Read the model definition and answer for the solid it produces. Units are mm, in the model's axes. A direction names the side the tool comes from. Coordinates: 2 decimals unless noted, no trailing zeros. Loops run counter-clockwise (first coordinate to the right, second up) from the corner with the lowest first, then second, coordinate; pieces in that order, holes last.
Autodesk Inventor part; units mm, degrees
ref_plane "YZ Plane" through (0, 0, 0) normal (1, 0, 0) x (0, 1, 0)
ref_plane "XZ Plane" through (0, 0, 0) normal (0, 1, 0) x (-1, 0, 0)
ref_plane "XY Plane" through (0, 0, 0) normal (0, 0, 1) x (1, 0, 0)
sketch "Sketch1" plane through (0, 0, 0) normal (0, 0, 1) x (1, 0, 0)
  line L0 (0, 0) -> (45.72, 0)
  line L1 (45.72, 0) -> (45.72, 34.29)
  line L2 (0, 0) -> (0, 82.169) construction
  line L3 (45.72, 34.29) -> (0, 82.169)
  line L4 (0, 0) -> (-45.72, 0)
  line L5 (-45.72, 0) -> (-45.72, 34.29)
  line L6 (-45.72, 34.29) -> (0, 82.169)
  dimension "d0" = 82.169
  dimension "d1" = 45.72
  dimension "d2" = 34.29
extrude "Extrusion1" add sketch "Sketch1" against normal blind 3.175
sketch "Sketch2" plane through (0, 0, 0) normal (0, 0, 1) x (1, 0, 0)
  line L0 (-45.72, 0) -> (-45.72, 34.29)
  line L1 (-45.72, 0) -> (45.72, 0)
  line L2 (45.72, 0) -> (45.72, 3.175)
  line L3 (45.72, 3.175) -> (-45.72, 3.175)
  line L4 (-45.72, 3.175) -> (-45.72, 0)
  point P0 (0, 0)
  dimension "d5" = 3.175
extrude "Extrusion2" add sketch "Sketch2" along normal blind 20.32
sketch "Sketch3" plane through (0, 0, 0) normal (0, 0, 1) x (1, 0, 0)
  circle A0 centre (0, 34.925) radius 15.113
  line L0 (-45.72, 0) -> (45.72, 0)
  point P0 (0, 0)
  dimension "d8" = 30.226
  dimension "d9" = 34.925
extrude "Extrusion3" cut sketch "Sketch3" against normal through all
properties part number "rsSnowBlowerMount"
Item 1: Determine the mould class of faces 1 (the face through (-23.18, 57.894, -1.565)), 2 (the face through (-11, 23, -3.175)), 3 (the face through (-11.14, 45.14, -1.57)), 4 (the face through (1, 0, 9)) for opening direction Y: released by +Y, released by -Y, zero draft, split by the parting line, or undercut.
Numbers:
face 1: released by +Y
face 2: zero draft
face 3: undercut
face 4: released by -Y
Item 2: A cutting plane is placed at C-C on y = 45.5. Determine the outline of the cut face in (x, z) (1 decimal), then the cut area to 3 significant figures.
Numbers:
outline: (-35, -3.2) - (-10.8, -3.2) - (-10.8, 0) - (-35, 0) - close; (10.8, -3.2) - (35, -3.2) - (35, 0) - (10.8, 0) - close
area: 154 mm2
Item 3: A cutting plane is placed at A-A on y = 31. Determine the outline of the cut face in (x, z) (3 decimals), then the cut area to 3 significant figures.
Numbers:
outline: (-45.72, -3.175) - (-14.594, -3.175) - (-14.594, 0) - (-45.72, 0) - close; (14.594, -3.175) - (45.72, -3.175) - (45.72, 0) - (14.594, 0) - close
area: 198 mm2
Item 4: Given pin 1 (6 mm diameter, centred on x = -8.5, y = 48, fed in from +Z); pin 2 (12 mm diameter, centred on x = -10.5, z = 15, fed in from +Y) (3 decimals), each flat-ended and moving along its own axis, determine where each tip first touches the part or whether it passes through.
Numbers:
pin 1: stops at z = 0
pin 2: stops at y = 3.175
Item 5: A cutting plane is placed at B-B on x = -10.5. Determine the outline of the cut face in (y, z) (3 decimals).
Numbers:
outline: (0, -3.175) - (24.055, -3.175) - (24.055, 0) - (3.175, 0) - (3.175, 20.32) - (0, 20.32) - close; (45.795, -3.175) - (71.173, -3.175) - (71.173, 0) - (45.795, 0) - close
Item 6: Which of the six approach directions +Z, -Z, +X, -X, +Y, -Y give full straight-line access (tool end or side, diameter ignored) to faces 5 (the face through (-1, 2, 20.32)), 6 (the face through (1, 3.175, 10))?
Numbers:
face 5: +Z, +X, -X, +Y, -Y
face 6: +Z, +X, -X, +Y
Item 7: A cutting plane is placed at D-D on x = -23.5. Determine the outline of the cut face in (y, z) (3 decimals).
Numbers:
outline: (0, -3.175) - (57.559, -3.175) - (57.559, 0) - (3.175, 0) - (3.175, 20.32) - (0, 20.32) - close
